Check sheet for the drawn part. Datum: minimum x, y, z corner. Units: mm. Coordinates: 2 decimals unless noted, no trailing zeros. Order: outer loops, then holes, each group sorted by start corner. A loop starts at its lowest first (then second) coordinate and runs counter-clockwise, first axis right, second up. Notation, with made-up numbers: M 32.5,86 L 61.5,86 A23 ccw 61.5,103 Z; hole C 12,72 d3. An arc over 180 degrees is marked long. Answer in a Markdown table with one row per item. Add a question column.
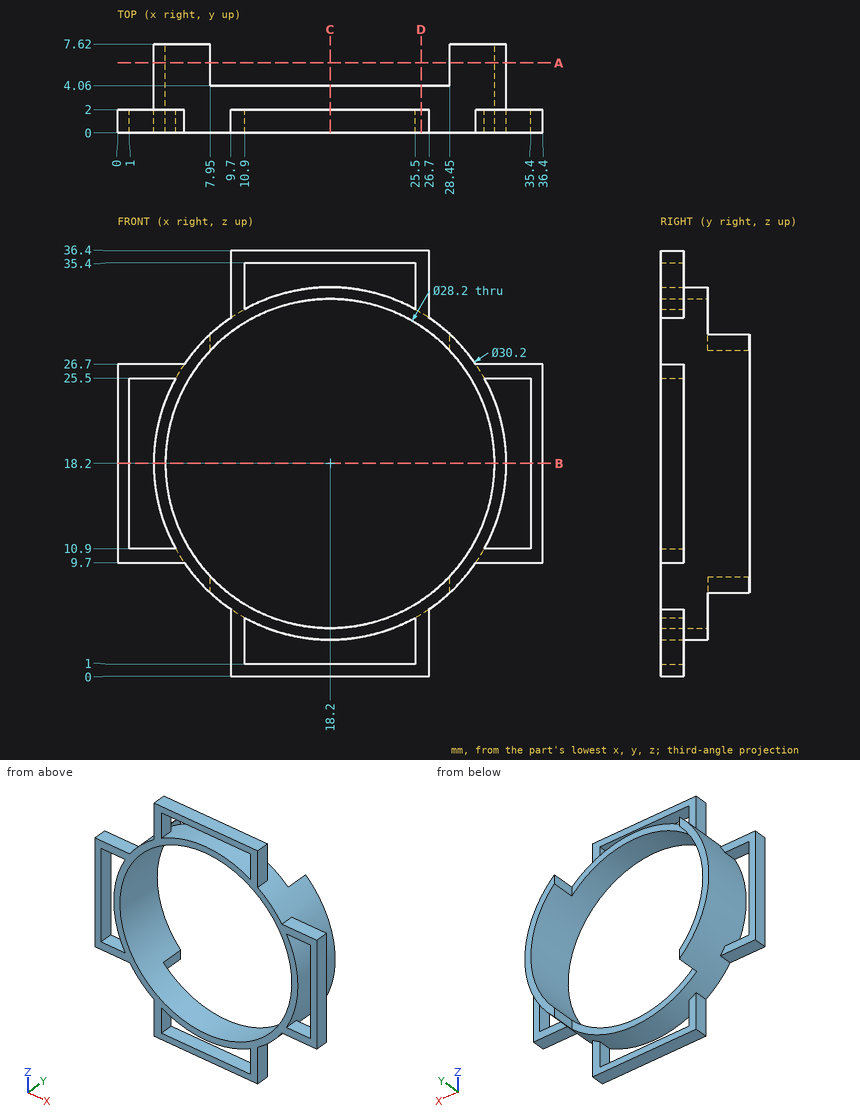
1. Go/stop test with flat-tipped pins: pin 1 Ø2 at (x, y) = (7.5, 4) entering from -Z; pin 2 Ø1.6 at (x, y) = (3, 0.5) entering from +Z; pin 3 Ø1.1 at (y, z) = (6, 8) entering from +X. Record where each tip stops, or that it passes through.
2. Section check D-D on x = 26. Enter the section's corners in (y, z), then the cut area to 3 significant figures.
3. Section check C-C on x = 18.2. Enter the section's corners in (y, z), then the cut area to 3 significant figures.
4. Section check A-A on y = 6. Enter the section's corners in (x, z).
5. Scan lines: line 1 (X direction, y = 7, z = 18.5); line 2 (X direction, y = 0.5, z = 12.5); line 3 (X direction, y = 6, z = 13). Record each from-to range of solid material in increasing order.
6. Section check B-B on z = 18.2. Enter the section's corners in (x, y), then the cut area to 3 significant figures.
Result sheet:
| question | item | result |
|---|---|---|
| 1 | pin 1 | z = 6.63 |
| 1 | pin 2 | z = 26.7 |
| 1 | pin 3 | x = 29.81 |
| 2 | outline | M 0,0 L 2,0 L 2,5.27 L 4.06,5.27 L 4.06,6.45 L 0,6.45 Z; M 0,29.95 L 4.06,29.95 L 4.06,31.13 L 2,31.13 L 2,36.4 L 0,36.4 Z |
| 2 | area | 30.7 mm^2 |
| 3 | outline | M 0,0 L 2,0 L 2,1 L 0,1 Z; M 0,3.1 L 4.06,3.1 L 4.06,4.1 L 0,4.1 Z; M 0,32.3 L 4.06,32.3 L 4.06,33.3 L 0,33.3 Z; M 0,35.4 L 2,35.4 L 2,36.4 L 0,36.4 Z |
| 3 | area | 12.1 mm^2 |
| 4 | outline | M 7.95,7.11 L 7.95,8.52 A14.1 cw 7.95,27.88 L 7.95,29.29 A15.1 ccw Z; M 28.45,7.11 A15.1 ccw 28.45,29.29 L 28.45,27.88 A14.1 cw 28.45,8.52 Z |
| 5 | line 1 | 3.1 to 4.1, 32.3 to 33.3 |
| 5 | line 2 | 0 to 1, 4.22 to 5.3, 31.1 to 32.18, 35.4 to 36.4 |
| 5 | line 3 | 4.02 to 5.09, 31.31 to 32.38 |
| 6 | outline | M 0,0 L 1,0 L 1,2 L 0,2 Z; M 3.1,0 L 4.1,0 L 4.1,7.62 L 3.1,7.62 Z; M 32.3,0 L 33.3,0 L 33.3,7.62 L 32.3,7.62 Z; M 35.4,0 L 36.4,0 L 36.4,2 L 35.4,2 Z |
| 6 | area | 19.2 mm^2 |
